from build123d import *

# Parameters (mm, degrees)
BOSS_EXTRUDE1_DEPTH = 60
SKETCH2_W           = 30
SKETCH2_H           = 107.13499281
BOSS_EXTRUDE2_DEPTH = 5
SKETCH3_W           = 80
SKETCH3_H           = 30
BOSS_EXTRUDE3_DEPTH = 5
BOSS_EXTRUDE4_DEPTH = 5
CUT_EXTRUDE2_DEPTH  = 5
SKETCH7_R           = 2.75
CUT_EXTRUDE3_DEPTH  = 178.183520676
SKETCH8_W           = 10
SKETCH8_H           = 6
SKETCH8_W_2         = 6
SKETCH8_H_2         = 10
CUT_EXTRUDE4_DEPTH  = 178.183520676
SKETCH10_W          = 13
SKETCH10_H          = 13
CUT_EXTRUDE5_DEPTH  = 178.183520676


with BuildPart() as part:
    # Sketch1 → Boss-Extrude1 (new body)
    with BuildSketch(Plane(origin=(0, 0, 0), x_dir=(1, 0, 0), z_dir=(0, 1, 0))):
        Polygon((0, 0), (0, 100), (3, 100), (3, 3), (83, 3), (83, 100), (86, 100), (86, 0), align=None)
    extrude(amount=BOSS_EXTRUDE1_DEPTH)

    # Sketch2 → Boss-Extrude2 (add)
    with BuildSketch(Plane(origin=(0, 60, 0), x_dir=(1, 0, 0), z_dir=(0, 1, 0))):
        with Locations((98, 66.432503591)):
            Rectangle(SKETCH2_W, SKETCH2_H)
        with Locations((-12, 66.432503591)):
            Rectangle(SKETCH2_W, SKETCH2_H)
    extrude(amount=BOSS_EXTRUDE2_DEPTH)

    # Sketch3 → Boss-Extrude3 (add)
    with BuildSketch(Plane(origin=(0, 65, 0), x_dir=(1, 0, 0), z_dir=(0, 1, 0))):
        with Locations((43, 104.999999996)):
            Rectangle(SKETCH3_W, SKETCH3_H)
    extrude(amount=-BOSS_EXTRUDE3_DEPTH)

    # Sketch5 → Boss-Extrude4 (add)
    with BuildSketch(Plane(origin=(0, 60, 0), x_dir=(1, 0, 0), z_dir=(0, 1, 0))):
        Polygon((0, 12.865007186), (0, 0), (86, 0), (86, 12.865007186), (83, 12.865007186), (83, 3), (3, 3), (3, 12.865007186), align=None)
    extrude(amount=BOSS_EXTRUDE4_DEPTH)

    # Sketch6 → Cut-Extrude2 (cut)
    with BuildSketch(Plane.XY):
        with BuildLine():
            Line((8, 0), (78, 0))
            ThreePointArc((78, 0), (43, 35), (8, 0))
        make_face()
    extrude(amount=-CUT_EXTRUDE2_DEPTH, mode=Mode.SUBTRACT)

    # Sketch7 → Cut-Extrude3 (cut, through all)
    with BuildSketch(Plane(origin=(0, 65, 0), x_dir=(1, 0, 0), z_dir=(0, 1, 0))):
        with Locations(Location((-12, 22.865007186, 0), (0, 0, 270))):
            Circle(SKETCH7_R)
        with Locations(Location((23, 104.999999996, 0), (0, 0, 270))):
            Circle(SKETCH7_R)
        with Locations(Location((98, 22.865007186, 0), (0, 0, 270))):
            Circle(SKETCH7_R)
    extrude(amount=-CUT_EXTRUDE3_DEPTH, mode=Mode.SUBTRACT)

    # Sketch8 → Cut-Extrude4 (cut, through all)
    with BuildSketch(Plane(origin=(0, 65, 0), x_dir=(1, 0, 0), z_dir=(0, 1, 0))):
        with Locations((-12, 52.499999996)):
            Rectangle(SKETCH8_W, SKETCH8_H)
        with Locations((35.581142125, 104.999999996)):
            Rectangle(SKETCH8_W_2, SKETCH8_H_2)
    extrude(amount=-CUT_EXTRUDE4_DEPTH, mode=Mode.SUBTRACT)

    # Sketch10 → Cut-Extrude5 (cut, through all)
    with BuildSketch(Plane(origin=(0, 65, 0), x_dir=(1, 0, 0), z_dir=(0, 1, 0))):
        with Locations((98, 47.865007186)):
            Rectangle(SKETCH10_W, SKETCH10_H)
    extrude(amount=-CUT_EXTRUDE5_DEPTH, mode=Mode.SUBTRACT)


solid = part.part
Could you check a few things on this model? Use its own coordinates, in mm. A direction names the side the tool comes from. Round coordinates to 2 decimals unless told otherwise and drop trailing zeros. Loops run counter-clockwise (first coordinate to the right, second up) from the corner with the lowest first, then second, coordinate; pieces in that order, holes last. Notation, with made-up numbers: (-39, -34.5) -> (12, -34.5) arc R19 ccw to (12, -23.5) -> close; hole circle Ø5 at (73, 40). An arc over 180 degrees is marked (long way). Use CSV: the item, a comma, the result in double quotes.
(1) Suppose I cut it at B-B on z = -18. Write out the boundary of the cut face in (x, y), plus the area to 3 significant figures.
Return value:
outline,"(-27, 60) -> (0, 60) -> (0, 0) -> (3, 0) -> (3, 65) -> (-27, 65) -> close; (83, 0) -> (86, 0) -> (86, 60) -> (113, 60) -> (113, 65) -> (83, 65) -> close"
area,"660 mm²"
(2) Suppose I cut it at A-A on x = -12. Write out the boundary of the cut face in (y, z) (3 decimals), plus the area to 3 significant figures.
Return value:
outline,"(60, -120) -> (65, -120) -> (65, -55.5) -> (60, -55.5) -> close; (60, -49.5) -> (65, -49.5) -> (65, -25.615) -> (60, -25.615) -> close; (60, -20.115) -> (65, -20.115) -> (65, -12.865) -> (60, -12.865) -> close"
area,"478 mm²"
(3) Suppose I cut it at D-D on x = 67.5. Write out the boundary of the cut face in (y, z) (3 decimals).
Return value:
outline,"(24.995, -3) -> (65, -3) -> (65, 0) -> (24.995, 0) -> close; (60, -120) -> (65, -120) -> (65, -90) -> (60, -90) -> close"
(4) For faces 1 (the flat face through (99, 62, -12.865)), 2 (the flat face through (1, 30, -100)), 3 (the flat face through (-14, 62, -12.865)), 4 (the flat face through (42, 39, 0)), 5 (the flat face through (-7, 63, -52)), which set-ups out of +Z, -Z, +X, -X, +Y, -Y let a thin tool reach every point of the face, with its end or its side?
Return value:
face 1,"+Z, +X, +Y, -Y"
face 2,"-Z, +X, -X, -Y"
face 3,"+Z, -X, +Y, -Y"
face 4,"+Z, +X, -X, +Y, -Y"
face 5,"+Y, -Y"
(5) If we mould it in two halves opening along Z, with no side actions, what happens to faces 6 (the flat face through (42, 65, -101)), 7 (the flat face through (42, 63, -120)), 8 (the flat face through (36, 63, -100))? For each: +Z half, -Z half, draft (parallel to the pull), parting line (faces both ways), or undercut.
Return value:
face 6,"draft"
face 7,"-Z half"
face 8,"undercut"
(6) If I drill on probe 1 along X at (y, z) = (63.05, -105); probe 2 along X at (y, z) = (41, -22.5); probe 3 along Z at (x, y) = (53.5, 59), over which ranges is the centre line in solid material (lowest first)? Write a range as [from, to].
Return value:
probe 1,"x = [-27, 20.25], [25.75, 32.58], [38.58, 113]"
probe 2,"x = [0, 3], [83, 86]"
probe 3,"z = [-3, 0]"
(7) Will these pins go through, and if not, where does the flat tip stop? pin 1 Ø0.9 at (x, y) = (1.5, 21) entering from -Z; pin 2 Ø8 at (x, y) = (37.5, 43.5) entering from -Z; pin 3 Ø8 at (y, z) = (41.5, -54.5) entering from -X; pin 4 Ø3 at (x, y) = (-2.5, 22) entering from +Z.
Return value:
pin 1,"stops at z = -100"
pin 2,"stops at z = -3"
pin 3,"stops at x = 0"
pin 4,"passes through"
(8) Suppose I cut it at C-C on z = -105. Write out the boundary of the cut face in (x, y).
Return value:
outline,"(-27, 60) -> (20.25, 60) -> (20.25, 65) -> (-27, 65) -> close; (25.75, 60) -> (32.58, 60) -> (32.58, 65) -> (25.75, 65) -> close; (38.58, 60) -> (113, 60) -> (113, 65) -> (38.58, 65) -> close"
